Check sheet for the modelled part. Datum: model origin and axes. Units: mm. A direction names the side the tool comes from. Round coordinates to 2 decimals unless told otherwise and drop trailing zeros. Write each loop counter-clockwise with the first axis right and the second up, starting at its lowest first coordinate (ties: lowest second). Pieces come first, ordered by that corner, then holes. Notation, with made-up numbers: M 12,34.25 L 48,34.25 A6 ccw 48,43.25 Z; hole C -5,33 d9. An arc over 180 degrees is marked long. One line per item, written item: value.
from build123d import *

# Parameters (mm, degrees)
SKETCH1_W           = 250
SKETCH1_H           = 150
BOSS_EXTRUDE1_DEPTH = 140
SKETCH2_W           = 209.504921958
SKETCH2_H           = 122.211204476
CUT_EXTRUDE1_DEPTH  = 130


with BuildPart() as part:
    # Sketch1 → Boss-Extrude1 (new body)
    with BuildSketch(Plane(origin=(0, 0, 0), x_dir=(1, 0, 0), z_dir=(0, 1, 0))):
        Rectangle(SKETCH1_W, SKETCH1_H)
    extrude(amount=BOSS_EXTRUDE1_DEPTH)

    # Sketch2 → Cut-Extrude1 (cut)
    with BuildSketch(Plane(origin=(0, 140, 0), x_dir=(1, 0, 0), z_dir=(0, 1, 0))):
        Rectangle(SKETCH2_W, SKETCH2_H)
    extrude(amount=-CUT_EXTRUDE1_DEPTH, mode=Mode.SUBTRACT)


solid = part.part
Q1. Depth check by flat-ended pin: P1, Ø6, axis at x = 31, z = 22.5, coming from the +Y side. Enter the tip coordinate at first touch or a pass-through.
Completed:
P1: y = 10
Q2. Scan lines: line 1 (X direction, y = 104, z = 55.5); line 2 (Z direction, x = 67.5, y = 39.5); line 3 (Y direction, x = -83.5, z = -48.5). Record each from-to range of solid material in increasing order. Write a range as [from, to].
Completed:
line 1: [-125, -104.75], [104.75, 125]
line 2: [-75, -61.11], [61.11, 75]
line 3: [0, 10]
Q3. Sectioned sample at C-C on x = 49.5. Enter the section's corners in (y, z), and give its area (3 significant figures).
Completed:
outline: M 0,-75 L 140,-75 L 140,-61.11 L 10,-61.11 L 10,61.11 L 140,61.11 L 140,75 L 0,75 Z
area: 5,110 mm^2
Q4. Sectioned sample at B-B on z = 58.5. Enter the section's corners in (x, y).
Completed:
outline: M -125,0 L 125,0 L 125,140 L 104.75,140 L 104.75,10 L -104.75,10 L -104.75,140 L -125,140 Z
Q5. Access from +Z, -Z, +X, -X, +Y, -Y to the whole of each face (thin tool, end or side, straight path). Record for faces 5 (the flat face through (-2, 0, -1)), 6 (the flat face through (-104.752, 76, 1)).
Completed:
face 5: +Z, -Z, +X, -X, -Y
face 6: +Y
Q6. Draft check along Z on faces 1 (the flat face through (-125, 69, 1)), 2 (the flat face through (-1, 76, -61.106)), 3 (the flat face through (-1, 76, 61.106)), 4 (the flat face through (-2, 69, -75)). Enter one of: pulls with the +Z half, pulls with the -Z half, needs draft (parallel to the pull), parting line crosses it, or undercut.
Completed:
face 1: needs draft
face 2: undercut
face 3: undercut
face 4: pulls with the -Z half
Q7. Sectioned sample at A-A on y = 131. Enter the section's corners in (x, z), and give its area (3 significant figures).
Completed:
outline: M -125,-75 L 125,-75 L 125,75 L -125,75 Z; hole M -104.75,-61.11 L 104.75,-61.11 L 104.75,61.11 L -104.75,61.11 Z
area: 11,900 mm^2
